Part model, mm, in its own coordinate system. A direction names the side the tool comes from. Give positions to 0.01 mm unless a question says otherwise; leave off trailing zeros. Order: outer loops, then holes, each group sorted by start corner. A loop starts at its lowest first (then second) coordinate and runs counter-clockwise, first axis right, second up. Notation, with made-up numbers: (79, 81) -> (115, 81) arc R26 ccw to (115, 106) -> close; hole circle Ø9 at (40, 77). An arc over 180 degrees is marked (long way). Write item = value, one per line. Start each with the question number.
Item 1: Band-saw the part on A-A on x = -1.05. Write the cut outline in (y, z) (3 decimals).
Item 2: Pull direction Y, two halves, no side cores. Call faces 3 (the face through (0, 10.085, 88)), 4 (the face through (0, -10.085, 88)), 5 (the face through (0, 0, 0)), 6 (the face through (-0.02, -0.03, 65.67)): +Y half, -Y half, draft (parallel to the pull), parting line (faces both ways), or undercut.
Item 3: Tool access for faces 1 (the face through (0, -1.415, 80)), 2 (the face through (1.588, 2, 89)): list every direction of +Z, -Z, +X, -X, +Y, -Y with a clear straight run to the whole face (end or side of a thin tool).
Item 4: Drill centre lines: line 1 along Y through (x, z) = (0.2, 170.08) (3 decimals); line 2 along Z through (x, y) = (0.5, 0.75); line 3 along Z through (x, y) = (-0.85, -9). Where is each one in solid material? Low to high.
Item 5: Flat gauge pin, fed straight in: P1, Ø3.5, axis at y = 0, z = 170.08, coming from the -X side. Where does the tip first touch, or does it go through?
```python
from build123d import *

# Parameters (mm, degrees)
SKETCH1_W           = 3.175
SKETCH1_H           = 20.17
BOSS_EXTRUDE1_DEPTH = 180.17
SKETCH6_R           = 1.415
CUT_EXTRUDE1_DEPTH  = 4.175
FILLET1_R           = 2.5
CUT_EXTRUDE3_DEPTH  = 10


with BuildPart() as part:
    # Sketch1 → Boss-Extrude1 (new body)
    with BuildSketch(Plane.XY):
        Rectangle(SKETCH1_W, SKETCH1_H)
    extrude(amount=BOSS_EXTRUDE1_DEPTH)

    # Sketch6 → Cut-Extrude1 (cut, through all)
    with BuildSketch(Plane(origin=(1.5875, 0, 0), x_dir=(0, 0, -1), z_dir=(1, 0, 0))):
        with Locations((-170.08, 0)):
            Circle(SKETCH6_R)
    extrude(amount=-CUT_EXTRUDE1_DEPTH, mode=Mode.SUBTRACT)

    # Fillet1
    fillet1_edges = [part.edges().sort_by_distance(p)[0] for p in [
        (0, -10.085, 180.17),
        (0, 10.085, 180.17),
    ]]
    fillet(fillet1_edges, radius=FILLET1_R)

    # Sketch7 → Cut-Extrude3 (cut)
    with BuildSketch(Plane.ZY.offset(1.5875)):
        with BuildLine():
            Line((67.085, 1.415), (93.085, 1.415))
            ThreePointArc((93.085, 1.415), (94.5, 0), (93.085, -1.415))
            Line((93.085, -1.415), (67.085, -1.415))
            ThreePointArc((67.085, -1.415), (65.67, 0), (67.085, 1.415))
        make_face()
    extrude(amount=-CUT_EXTRUDE3_DEPTH, mode=Mode.SUBTRACT)


solid = part.part
```
Values found:
q1.outline = (-10.085, 0) -> (10.085, 0) -> (10.085, 177.67) arc R2.5 ccw to (7.585, 180.17) -> (-7.585, 180.17) arc R2.5 ccw to (-10.085, 177.67) -> close; hole (-1.415, 67.085) arc R1.415 ccw to (1.415, 67.085) -> (1.415, 93.085) arc R1.415 ccw to (-1.415, 93.085) -> close; hole circle Ø2.83 at (0, 170.08)
q2.face_3 = +Y half
q2.face_4 = -Y half
q2.face_5 = draft
q2.face_6 = undercut
q3.face_1 = +X, -X
q3.face_2 = +Z, -Z, +X, +Y, -Y
q4.line_1 = -10.085 to -1.415, 1.415 to 10.085
q4.line_2 = 0 to 65.89, 94.28 to 168.88, 171.28 to 180.17
q4.line_3 = 0 to 179.73
q5.P1 = -1.59
